Geometry check sheet. Reference: the model listing, model coordinates, mm. A direction names the side the tool comes from. Coordinates: 2 decimals unless noted, no trailing zeros. Write each loop counter-clockwise with the first axis right and the second up, starting at its lowest first coordinate (ties: lowest second). Pieces come first, ordered by that corner, then holes. Notation, with made-up numbers: (57, 63) -> (93, 63) arc R20 cw to (93, 100) -> close; hole circle Ø10 at (-9, -34). An arc over 180 degrees is marked (long way). Use a Markdown table: item, result.
```python
from build123d import *

# Parameters (mm, degrees)
SKETCH1_W           = 19.05
SKETCH1_H           = 19.05
BOSS_EXTRUDE1_DEPTH = 50.8
SKETCH4_W           = 1.5875
SKETCH4_H           = 19.05
CUT_EXTRUDE1_DEPTH  = 29.21
CUT_EXTRUDE2_START  = -19.05
SKETCH5_R           = 6.35
CUT_EXTRUDE2_DEPTH  = 19.05
FILLET3_R           = 9.05
SKETCH6_R           = 1.5875
CUT_EXTRUDE3_DEPTH  = 19.05


with BuildPart() as part:
    # Sketch1 → Boss-Extrude1 (new body)
    with BuildSketch(Plane(origin=(0, 0, 0), x_dir=(1, 0, 0), z_dir=(0, 1, 0))):
        Rectangle(SKETCH1_W, SKETCH1_H)
    extrude(amount=BOSS_EXTRUDE1_DEPTH)

    # Sketch4 → Cut-Extrude1 (cut)
    with BuildSketch(Plane(origin=(0, 50.8, 0), x_dir=(1, 0, 0), z_dir=(0, 1, 0))):
        Rectangle(SKETCH4_W, SKETCH4_H)
    extrude(amount=-CUT_EXTRUDE1_DEPTH, mode=Mode.SUBTRACT)

    # Sketch5 → Cut-Extrude2 (cut)
    with BuildSketch(Plane.XY.offset(9.525).offset(CUT_EXTRUDE2_START)):
        with Locations((0, 30.48)):
            Circle(SKETCH5_R)
    extrude(amount=CUT_EXTRUDE2_DEPTH, mode=Mode.SUBTRACT)

    # Fillet3
    fillet3_edges = [part.edges().sort_by_distance(p)[0] for p in [
        (0, 0, 9.525),
        (0, 0, -9.525),
    ]]
    fillet(fillet3_edges, radius=FILLET3_R)

    # Sketch6 → Cut-Extrude3 (cut)
    with BuildSketch(Plane(origin=(9.525, 0, 0), x_dir=(0, 0, -1), z_dir=(1, 0, 0))):
        with Locations((0.047497924, 45.720222057)):
            Circle(SKETCH6_R)
        with Locations((0.368108908, 11.431720944)):
            Circle(SKETCH6_R)
    extrude(amount=-CUT_EXTRUDE3_DEPTH, mode=Mode.SUBTRACT)


solid = part.part
```
Item 1: Section check A-A on x = -4.75. Count the separate pieces of the cut face and the enclosed holes in it, then the cut area to 3 significant figures.
Answer block:
| item | result |
|---|---|
| separate pieces | 2 |
| enclosed holes | 2 |
| area | 756 mm^2 |
Item 2: Depth check by flat-ended pin: P1, Ø1.9, axis at y = 45.72, z = -0.05, coming from the -X side. Enter the tip coordinate at first touch or a pass-through.
Answer block:
| item | result |
|---|---|
| P1 | passes through |
Item 3: Mould release check, pull along Z, two halves, no side actions. Record for faces 4 (the flat face through (-4, 25, -9.525)), 5 (the cylindrical face through (6.35, 30.35, -0.13)), 6 (the cylindrical face through (0.133, 13.006, -0.161)): +Z half, -Z half, draft (parallel to the pull), parting line (faces both ways), or undercut.
Answer block:
| item | result |
|---|---|
| face 4 | -Z half |
| face 5 | draft |
| face 6 | undercut |
Item 4: Section check B-B on y = 22.5. Record the boundary of the cut face in (x, z) (3 decimals).
Answer block:
| item | result |
|---|---|
| outline | (-9.525, -9.525) -> (-0.794, -9.525) -> (-0.794, 9.525) -> (-9.525, 9.525) -> close; (0.794, -9.525) -> (9.525, -9.525) -> (9.525, 9.525) -> (0.794, 9.525) -> close |
Item 5: Section check C-C on z = 5.5. Record the boundary of the cut face in (x, y) (3 decimals), then the cut area to 3 significant figures.
Answer block:
| item | result |
|---|---|
| outline | (-9.525, 1.523) -> (9.525, 1.523) -> (9.525, 50.8) -> (0.794, 50.8) -> (0.794, 36.78) arc R6.35 cw to (0.794, 24.18) -> (0.794, 21.59) -> (-0.794, 21.59) -> (-0.794, 24.18) arc R6.35 cw to (-0.794, 36.78) -> (-0.794, 50.8) -> (-9.525, 50.8) -> close |
| area | 786 mm^2 |
Item 6: Thickness scan on L1, parallel to X at y = 44, z = 5.5 (3 decimals); L2, parallel to Y at x = 5.5, z = -1; L3, parallel to Y at x = -8, z = -1.75. Record the ranges inside material, lowest first. Write a range as [from, to].
Answer block:
| item | result |
|---|---|
| L1 | x = [-9.525, -0.794], [0.794, 9.525] |
| L2 | y = [0.02, 9.98], [12.89, 27.31], [33.65, 44.45], [46.99, 50.8] |
| L3 | y = [0.09, 10.65], [12.21, 50.8] |
Item 7: Tool access check on faces 1 (the cylindrical face through (-6.35, 30.61, -0.13)), 2 (the flat face through (-5, 50.8, 0)), 3 (the flat face through (-0.794, 43.9, 0.1)). Record the directions out of +Z, -Z, +X, -X, +Y, -Y that give a thin tool (end or side, any length) a straight path to the whole face; none if there is none.
Answer block:
| item | result |
|---|---|
| face 1 | +Z, -Z |
| face 2 | +Z, -Z, +X, -X, +Y |
| face 3 | +Z, -Z, +Y |
